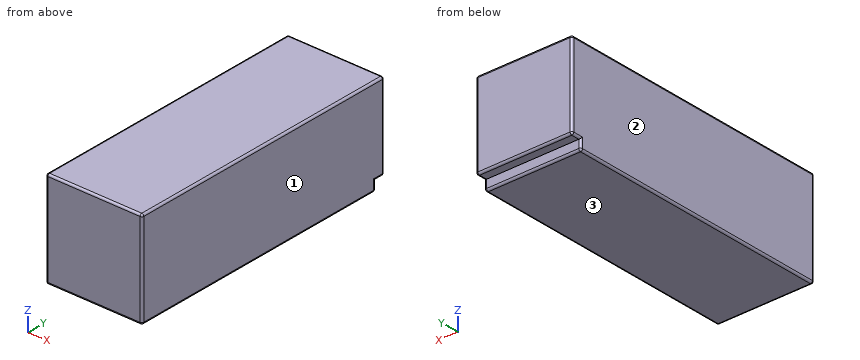
```python
from build123d import *

# Parameters (mm, degrees)
SKETCH1_W               = 48
SKETCH1_H               = 48
BOSS_EXTRUDE1_DEPTH     = 69.5
CUT_EXTRUDE1_DEPTH      = 78.345006303
CUT_EXTRUDE1_DEPTH_BACK = 78.345006303
SKETCH2_W               = 5
SKETCH2_H               = 5
FILLET1_R               = 1


with BuildPart() as part:
    # Sketch1 → Boss-Extrude1 (new, symmetric)
    with BuildSketch(Plane(origin=(0, 0, 0), x_dir=(1, 0, 0), z_dir=(0, 1, 0))):
        Rectangle(SKETCH1_W, SKETCH1_H)
    extrude(amount=BOSS_EXTRUDE1_DEPTH, both=True)

    # Sketch2 → Cut-Extrude1 (cut, two sides: drawn at the far end of the back side and taken through both)
    with BuildSketch(Plane(origin=(0, 0, 0), x_dir=(0, 0, -1), z_dir=(1, 0, 0)).offset(-CUT_EXTRUDE1_DEPTH_BACK)):
        with Locations((21.5, 67)):
            Rectangle(SKETCH2_W, SKETCH2_H)
    extrude(amount=CUT_EXTRUDE1_DEPTH + CUT_EXTRUDE1_DEPTH_BACK, mode=Mode.SUBTRACT)

    # Fillet1
    fillet1_edges = [part.edges().sort_by_distance(p)[0] for p in [
        (24, 69.5, 2.5),
        (-24, 69.5, 2.5),
        (-24, -2.5, -24),
        (24, -2.5, -24),
        (0, 64.5, -24),
        (-24, 64.5, -21.5),
        (-24, 67, -19),
        (0, 69.5, -19),
        (24, 67, -19),
        (24, 64.5, -21.5),
        (0, -69.5, -24),
        (24, -69.5, 0),
        (0, -69.5, 24),
        (-24, -69.5, 0),
        (24, 0, 24),
        (-24, 0, 24),
        (0, 69.5, 24),
    ]]
    fillet(fillet1_edges, radius=FILLET1_R)


solid = part.part
```
Part model, mm, in its own coordinate system. Face numbers are marked on the shaded views. Coordinates: 2 decimals unless noted, no trailing zeros. Order: outer loops, then holes, each group sorted by start corner. A loop starts at its lowest first (then second) coordinate and runs counter-clockwise, first axis right, second up. Notation, with made-up numbers: (46, 57.5) -> (73, 57.5) arc R28 ccw to (73, 82.5) -> close; hole circle Ø4 at (61.5, 82). An arc over 180 degrees is marked (long way). Put each result on its own line as item: value. Start each with the question number.
(1) Band-saw the part on A-A (z = -21). Give the cut face in (x, y).
(2) Mould opens along X. For the marked faces 1, 2 and 3 say: pulls with the +X half, pulls with the -X half, needs draft (parallel to the pull), parting line crosses it, or undercut.
(3) Pin check, flat tips, straight feed: pin 1 Ø1.2 at (x, z) = (9, -20.5) entering from +Y; pin 2 Ø3 at (x, y) = (3.5, 67) entering from -Z. Stop position of each tip, or through.
Determined:
1. outline: (-24, -68.5) arc R1 ccw to (-23, -69.5) -> (23, -69.5) arc R1 ccw to (24, -68.5) -> (24, 63.5) arc R1 ccw to (23, 64.5) -> (-23, 64.5) arc R1 ccw to (-24, 63.5) -> close
2. face 1: pulls with the +X half
2. face 2: pulls with the -X half
2. face 3: needs draft
3. pin 1: stops at y = 64.5
3. pin 2: stops at z = -19
